```python
from build123d import *

# Parameters (mm, degrees)
F0_R     = 3.175
F1_DEPTH = 3.175


with BuildPart() as f1:
    # F0 (on Front) → F1 (new body)
    with BuildSketch(Plane.XZ):
        with BuildLine():
            Line((20.588394, 20.031052), (-17.511606, 20.031052))
            ThreePointArc((-17.511606, 20.031052), (-26.491862, 16.311308), (-30.211606, 7.331052))
            Line((-30.211606, 7.331052), (-30.211606, -18.068948))
            ThreePointArc((-30.211606, -18.068948), (-26.491862, -27.049204), (-17.511606, -30.768948))
            Line((-17.511606, -30.768948), (20.588394, -30.768948))
            Line((20.588394, -30.768948), (20.588394, 20.031052))
        make_face()
        with Locations((-17.511606, -5.368948)):
            Circle(F0_R, mode=Mode.SUBTRACT)
    extrude(amount=F1_DEPTH)


solid = f1.part
```
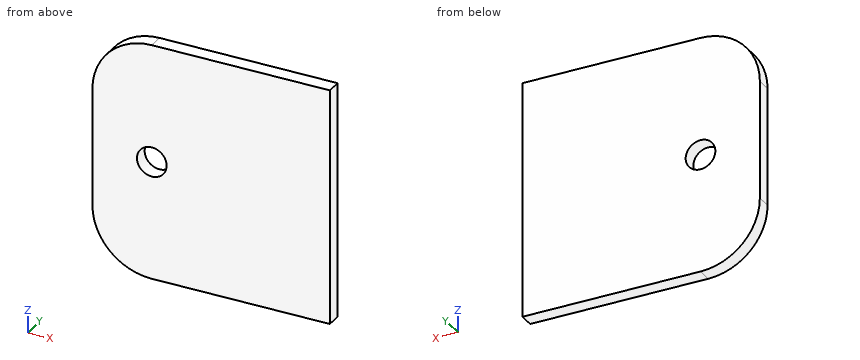
Verification items for the finished model (mm, model axes). Coordinates: 2 decimals unless noted, no trailing zeros. Order: outer loops, then holes, each group sorted by start corner. A loop starts at its lowest first (then second) coordinate and runs counter-clockwise, first axis right, second up. Notation, with made-up numbers: (77, 64.5) -> (103, 64.5) arc R18 cw to (103, 88.5) -> close; hole circle Ø9 at (-8, -0.75). An arc over 180 degrees is marked (long way). Put each result on its own line as item: value. Start each with the question number.
1) Cross-section at A-A (y = -1.75). Enter the section's corners in (x, z) (3 decimals), plus the area to 3 significant figures.
2) Cross-section at C-C (z = 12). Enter the section's corners in (x, y) (3 decimals).
3) Cross-section at B-B (z = -7). Enter the section's corners in (x, y) (3 decimals).
4) Material ranges on L1, parallel to X at y = -1.65, z = -6.5; L2, parallel to Z at x = -20, y = -2.4; L3, parallel to X at y = -0.4, z = 17, recorded low to high.
5) Cross-section at D-D (z = -27). Enter the section's corners in (x, y) (3 decimals).
Geometry check:
1. outline: (-30.212, -18.069) arc R12.7 ccw to (-17.512, -30.769) -> (20.588, -30.769) -> (20.588, 20.031) -> (-17.512, 20.031) arc R12.7 ccw to (-30.212, 7.331) -> close; hole circle Ø6.35 at (-17.512, -5.369)
1. area: 2,480 mm^2
2. outline: (-29.322, -3.175) -> (20.588, -3.175) -> (20.588, 0) -> (-29.322, 0) -> close
3. outline: (-30.212, -3.175) -> (-20.236, -3.175) -> (-20.236, 0) -> (-30.212, 0) -> close; (-14.788, -3.175) -> (20.588, -3.175) -> (20.588, 0) -> (-14.788, 0) -> close
4. L1: x = -30.21 to -20.48, -14.54 to 20.59
4. L2: z = -30.52 to -7.34, -3.4 to 19.78
4. L3: x = -25.75 to 20.59
5. outline: (-26.541, -3.175) -> (20.588, -3.175) -> (20.588, 0) -> (-26.541, 0) -> close
